from build123d import *

# Parameters (mm, degrees)
PAD_DEPTH     = 75
SKETCH001_R   = 24.4
SKETCH001_R_2 = 2.5
PAD001_DEPTH  = 75
SKETCH003_R   = 24.4
PAD002_DEPTH  = 5
SKETCH004_R   = 25.4
POCKET_DEPTH  = 3
PAD003_DEPTH  = 10
FILLET_R      = 7


with BuildPart() as part:
    # Sketch → Pad (new body)
    with BuildSketch(Plane.XY):
        with BuildLine():
            ThreePointArc((-29.848016, -3.015947), (29.920505, -2.182515), (-29.094406, 7.315431))
            ThreePointArc((-29.094406, 7.315431), (-29.072912, 3.034578), (-26.991574, -0.706304))
            Line((-26.991574, -0.706304), (-12.739759, -15.728805))
            ThreePointArc((-12.739759, -15.728805), (-11.4789, -15.911046), (-11.008743, -14.727014))
            Line((-11.008743, -14.727014), (-18.604437, 10.709188))
            ThreePointArc((-18.160969, 13.282665), (-18.684551, 12.047942), (-18.604437, 10.709188))
            ThreePointArc((-20.499669, -9.27435), (22.380035, -2.320351), (-18.160969, 13.282665))
            ThreePointArc((-20.499669, -9.27435), (-21.232479, -7.959372), (-22.173804, -6.784601))
            Line((-22.173804, -6.784601), (-26.991574, -1.706304))
            ThreePointArc((-26.991574, -1.706304), (-28.888073, -1.339771), (-29.848016, -3.015947))
        make_face()
    extrude(amount=PAD_DEPTH)

    # Sketch001 (on DatumPlane) → Pad001 (join)
    with BuildSketch(Plane.XY.offset(75)):
        with BuildLine():
            ThreePointArc((-28.4, -66.9), (0, -95.3), (28.4, -66.9))
            ThreePointArc((28.4, -66.9), (24.824987, -53.105798), (15, -42.784445))
            Line((15, -16.77051), (15, -42.784445))
            ThreePointArc((-15, -16.77051), (0, -22.5), (15, -16.77051))
            Line((-15, -16.77051), (-15, -42.784445))
            ThreePointArc((-15, -42.784445), (-24.824987, -53.105798), (-28.4, -66.9))
        make_face()
        with Locations((0, -66.9)):
            Circle(SKETCH001_R, mode=Mode.SUBTRACT)
        with Locations((-4, -32.5)):
            Circle(SKETCH001_R_2, mode=Mode.SUBTRACT)
        with Locations((4, -32.5)):
            Circle(SKETCH001_R_2, mode=Mode.SUBTRACT)
    extrude(amount=-PAD001_DEPTH)

    # Sketch003 (on DatumPlane) → Pad002 (join)
    with BuildSketch(Plane.XY.offset(75)):
        with Locations((0, -66.9)):
            Circle(SKETCH003_R)
    extrude(amount=-PAD002_DEPTH)

    # Sketch004 (on DatumPlane) → Pocket (cut)
    with BuildSketch(Plane(origin=(0, 0, 0), x_dir=(1, 0, 0), z_dir=(0, 0, -1))):
        with Locations((0, 66.9)):
            Circle(SKETCH004_R)
    extrude(amount=-POCKET_DEPTH, mode=Mode.SUBTRACT)

    # Sketch005 (on DatumPlane) → Pad003 (join)
    with BuildSketch(Plane(origin=(0, 0, 0), x_dir=(1, 0, 0), z_dir=(0, 0, -1))):
        with BuildLine():
            Line((-28.023442, -10.709188), (-18.160969, -13.282665))
            ThreePointArc((-18.160969, -13.282665), (15.109476, -16.671944), (15, 16.77051))
            Line((15, 16.77051), (15, 25.980762))
            ThreePointArc((-28.023442, -10.709188), (19.466397, -22.826725), (15, 25.980762))
        make_face()
    extrude(amount=PAD003_DEPTH)

    # Fillet
    fillet_edges = [part.edges().sort_by_distance(p)[0] for p in [
        (15.109476, 16.671944, -10),
        (-23.092205, 11.995927, -10),
        (15, -21.375636, -10),
    ]]
    fillet(fillet_edges, radius=FILLET_R)


solid = part.part
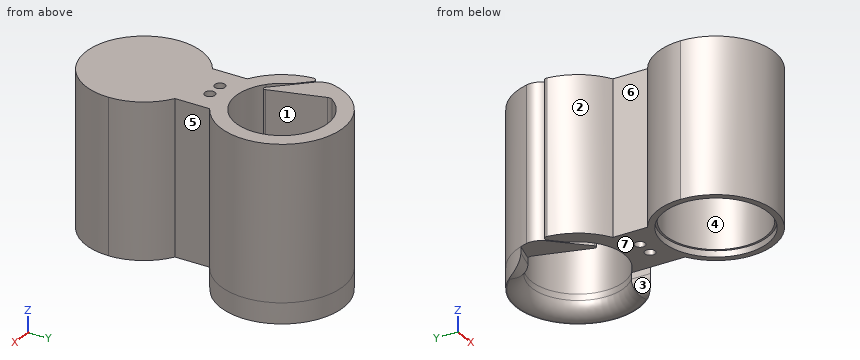
Geometry check sheet. Reference: the model listing, model coordinates, mm. Face numbers are marked on the shaded views. A direction names the side the tool comes from. Round coordinates to 2 decimals unless told otherwise and drop trailing zeros. Loops run counter-clockwise (first coordinate to the right, second up) from the corner with the lowest first, then second, coordinate; pieces in that order, holes last. Notation, with made-up numbers: (54.5, 16) -> (67.5, 16) arc R18 cw to (67.5, 27) -> close; hole circle Ø7 at (21, 23.5). An arc over 180 degrees is marked (long way). Answer as a JSON object with one key per item and string values. Group by question number.
Item 1: Cross-section at A-A, the plane y = -32.5. Record the cut outline in (x, z).
Item 2: Set-up check for the marked faces 1, 2, 3, 4 and 5: record each of +Z, -Z, +X, -X, +Y, -Y from which the full face is reachable in a straight line by a thin tool's end or side.
Item 3: Thickness scan on line 1 along Y through (x, z) = (0, 54); line 2 along Y through (x, z) = (-20.5, 62.5); line 3 along Y through (x, z) = (-7.5, 44). Record the ranges inside material, lowest first.
Item 4: Cross-section at B-B, the plane z = 19. Record the cut outline in (x, y), plus the area to 3 significant figures.
Item 5: Release check for a two-part mould opening along Y. For the marked faces 6 and 7 record: pulls with the +Y half, pulls with the -Y half, needs draft (parallel to the pull), parting line crosses it, or undercut.
Item 6: Cross-section at D-D, the plane x = 4. Count the separate pieces of the cut face and the enclosed holes in it, plus the area to 3 significant figures.
Item 7: Cross-section at C-C, the plane y = -59. Record the cut outline in (x, z).
Item 8: Depth check by flat-ended pin: pin 1 Ø8 at (x, y) = (22, -47.5) entering from -Z; pin 2 Ø15 at (x, y) = (4, -70.5) entering from -Z; pin 3 Ø8.5 at (y, z) = (-30.5, 19) entering from -X. Enter the tip coordinate at first touch or a pass-through.
Determined:
{
 "1": {"outline": "(-15, 0) -> (-6.5, 0) -> (-6.5, 75) -> (-15, 75) -> close; (-1.5, 0) -> (1.5, 0) -> (1.5, 75) -> (-1.5, 75) -> close; (6.5, 0) -> (15, 0) -> (15, 75) -> (6.5, 75) -> close"},
 "2": {"face 1": "+Z, -Z", "face 2": "+Z, -Z, -X", "face 3": "-Z, -X, -Y", "face 4": "-Z", "face 5": "+Z, -Z, +X"},
 "3": {"line 1": "y = -95.3 to -91.3, -42.5 to -22.5, 22.5 to 30", "line 2": "y = -86.55 to -80.13, -53.67 to -47.25, -21.9 to -9.27, -7.55 to 21.9", "line 3": "y = -94.29 to -90.12, -43.68 to -21.21, 21.21 to 29.05"},
 "4": {"outline": "(-29.85, -3.02) arc R30 ccw to (-15, -25.98) -> (-15, -42.78) arc R28.4 ccw (long way) to (28.4, -66.9) arc R28.4 ccw to (15, -42.78) -> (15, -25.98) arc R30 ccw (long way) to (-29.09, 7.32) arc R8.61 ccw to (-26.99, -0.71) -> (-12.74, -15.73) arc R1.03 ccw to (-11.01, -14.73) -> (-18.6, 10.71) arc R2.94 cw to (-18.16, 13.28) arc R22.5 cw (long way) to (-20.5, -9.27) arc R9.02 ccw to (-22.17, -6.78) -> (-26.99, -1.71) arc R1.66 ccw to start; hole circle Ø48.8 at (0, -66.9); hole circle Ø5 at (-4, -32.5); hole circle Ø5 at (4, -32.5)", "area": "2,330 mm²"},
 "5": {"face 6": "undercut", "face 7": "needs draft"},
 "6": {"separate pieces": "3", "enclosed holes": "0", "area": "2,350 mm²"},
 "7": {"outline": "(-27.28, 0) -> (-24.14, 0) -> (-24.14, 3) -> (-23.09, 3) -> (-23.09, 70) -> (23.09, 70) -> (23.09, 3) -> (24.14, 3) -> (24.14, 0) -> (27.28, 0) -> (27.28, 75) -> (-27.28, 75) -> close"},
 "8": {"pin 1": "stops at z = 0", "pin 2": "stops at z = 70", "pin 3": "stops at x = -15"}
}
